Source: three-view drawing plus pictorial views. Frame: mm from the lowest corner of the part. Coordinates: 2 decimals unless noted, no trailing zeros. Write each loop counter-clockwise with the first axis right and the second up, starting at its lowest first coordinate (ties: lowest second). Pieces come first, ordered by that corner, then holes. Notation, with made-up numbers: (-25.5, 77.25) - (-16.5, 77.25) arc R22 ccw to (-16.5, 98.25) - close; hole circle Ø1 at (28.25, 64). An arc over 180 degrees is marked (long way). Put each result on its own line as item: value.
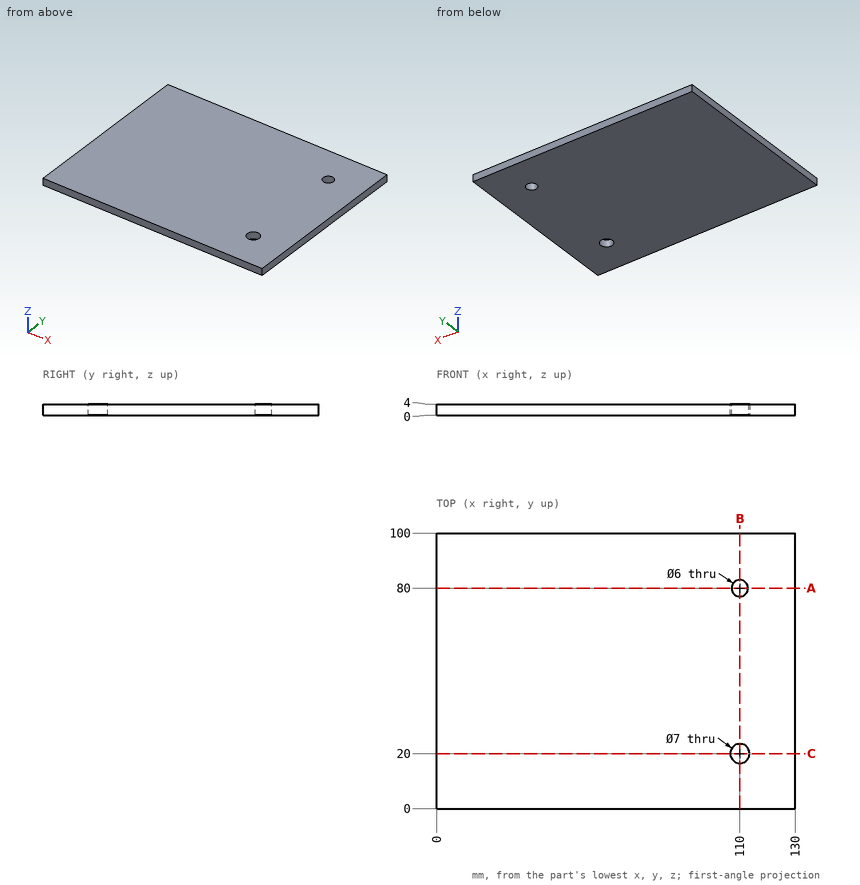
1. Section query B-B (x = 110). Return loops of the section in (y, z).
Answer below:
outline: (0, 0) - (16.5, 0) - (16.5, 4) - (0, 4) - close; (23.5, 0) - (77, 0) - (77, 4) - (23.5, 4) - close; (83, 0) - (100, 0) - (100, 4) - (83, 4) - close
2. Pin query (flat end, axial travel): pin 1 Ø3.5 at (x, y) = (110, 80) entering from +Z. Return the tip coordinate at first contact, or that it passes through.
Answer below:
pin 1: passes through
3. Section query C-C (y = 20). Return loops of the section in (x, z).
Answer below:
outline: (0, 0) - (106.5, 0) - (106.5, 4) - (0, 4) - close; (113.5, 0) - (130, 0) - (130, 4) - (113.5, 4) - close
4. Ray query, probe 1 along Y at (x, z) = (110, 1.5). Return the intervals inside material, ascending. Write a range as from..to.
Answer below:
probe 1: y = 0..16.5, 23.5..77, 83..100
5. Section query A-A (y = 80). Return loops of the section in (x, z).
Answer below:
outline: (0, 0) - (107, 0) - (107, 4) - (0, 4) - close; (113, 0) - (130, 0) - (130, 4) - (113, 4) - close
